Verification items for this drawing (mm, ordinates from the low corner). A direction names the side the tool comes from. Coordinates: 2 decimals unless noted, no trailing zeros. Write each loop counter-clockwise with the first axis right and the second up, starting at its lowest first coordinate (ties: lowest second). Pieces come first, ordered by that corner, then holes. Notation, with made-up numbers: (44.25, -32.5) -> (98.25, -32.5) arc R13 cw to (98.25, -7.5) -> close; hole circle Ø9 at (2.5, 82.25). An arc over 180 degrees is marked (long way). Use CSV: the item, a comma, the result in double quotes.
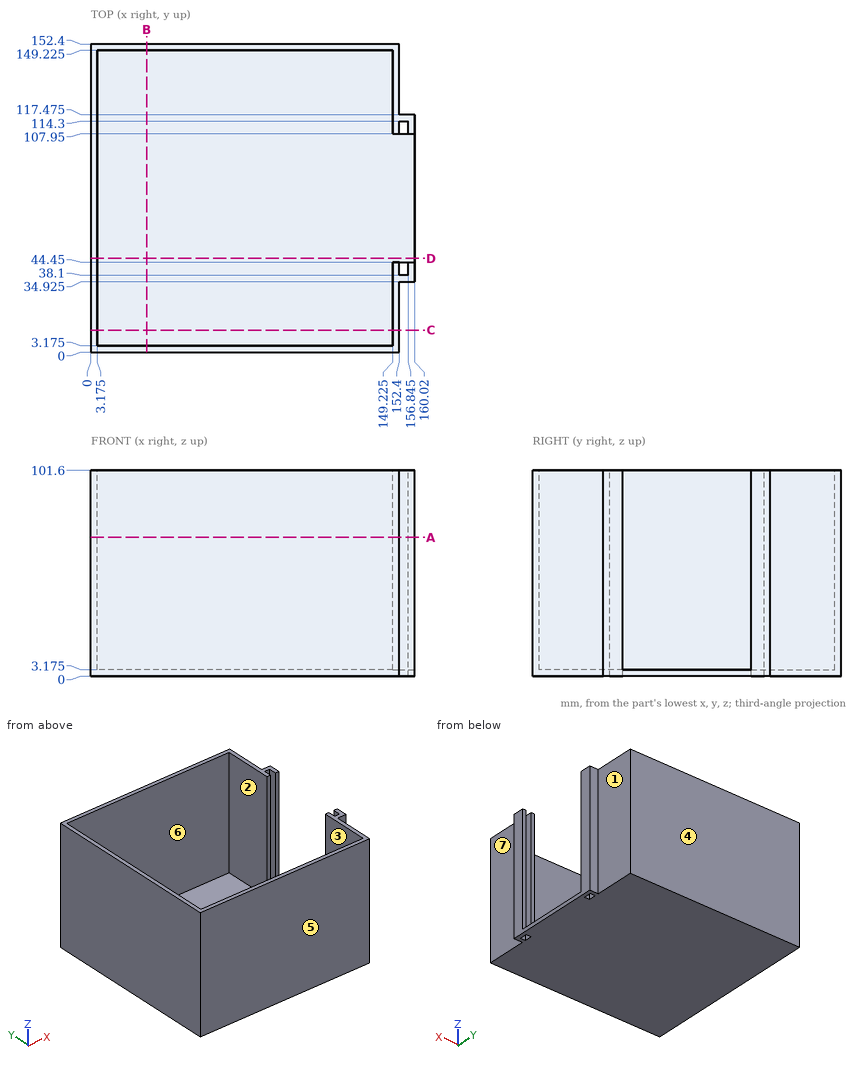
1) Cross-section at B-B (x = 27.5). Record the boundary of the cut face in (y, z) (3 decimals), plus the area to 3 significant figures.
Return value:
outline,"(0, 0) -> (152.4, 0) -> (152.4, 101.6) -> (149.225, 101.6) -> (149.225, 3.175) -> (3.175, 3.175) -> (3.175, 101.6) -> (0, 101.6) -> close"
area,"1,110 mm2"
2) Mould release check, pull along X, two halves, no side actions. Record for the marked faces 1, 2, 3 and 4: released by +X, released by -X, zero draft, split by the parting line, or undercut.
Return value:
face 1,"released by +X"
face 2,"undercut"
face 3,"undercut"
face 4,"zero draft"
3) Scan lines: L1, parallel to X at y = 25.5, z = 54 (3 decimals); L2, parallel to Z at x = 36, y = 54 (3 decimals). Record each from-to range of solid material in increasing order.
Return value:
L1,"0 to 3.175, 149.225 to 152.4"
L2,"0 to 3.175"
4) Set-up check for the marked faces 5, 6 and 7: record each of +Z, -Z, +X, -X, +Y, -Y from which the full face is reachable in a straight line by a thin tool's end or side.
Return value:
face 5,"+Z, -Z, +X, -X, -Y"
face 6,"+Z"
face 7,"+Z, -Z, +X, -Y"
5) Gauge pin test, flat ends, axial feed: pin 1 (1 mm diameter, centred on x = 154, z = 2, fed in from +Y) (3 decimals); pin 2 (1 mm diameter, centred on x = 93.5, y = 24, fed in from -Z); pin 3 (2.5 mm diameter, centred on x = 159, z = 31, fed in from -Y) (3 decimals); pin 4 (6 mm diameter, centred on x = 130.5, y = 19.5, fed in from +Z) (3 decimals). Record the tip position at first contact, or that the pin passes through.
Return value:
pin 1,"y = 117.475"
pin 2,"z = 0"
pin 3,"y = 34.925"
pin 4,"z = 3.175"
6) Cross-section at A-A (z = 68.5). Record the boundary of the cut face in (x, y) (3 decimals).
Return value:
outline,"(0, 0) -> (152.4, 0) -> (152.4, 34.925) -> (160.02, 34.925) -> (160.02, 44.45) -> (156.845, 44.45) -> (156.845, 38.1) -> (152.4, 38.1) -> (152.4, 44.45) -> (149.225, 44.45) -> (149.225, 3.175) -> (3.175, 3.175) -> (3.175, 149.225) -> (149.225, 149.225) -> (149.225, 107.95) -> (152.4, 107.95) -> (152.4, 114.3) -> (156.845, 114.3) -> (156.845, 107.95) -> (160.02, 107.95) -> (160.02, 117.475) -> (152.4, 117.475) -> (152.4, 152.4) -> (0, 152.4) -> close"
7) Cross-section at D-D (y = 46.5). Record the boundary of the cut face in (x, z) (3 decimals), plus the area to 3 significant figures.
Return value:
outline,"(0, 0) -> (160.02, 0) -> (160.02, 3.175) -> (3.175, 3.175) -> (3.175, 101.6) -> (0, 101.6) -> close"
area,"821 mm2"
